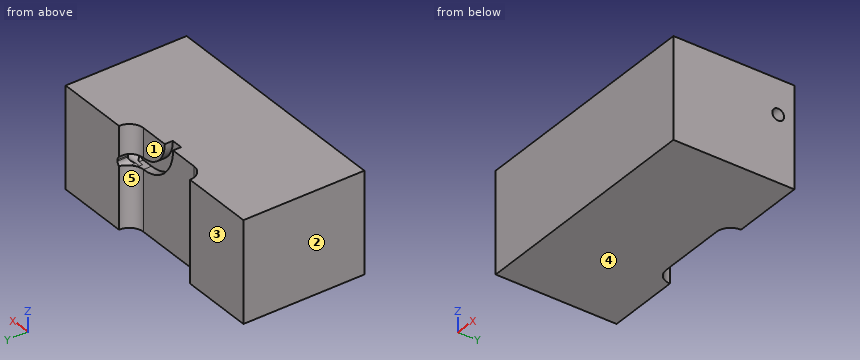
from build123d import *

# Parameters (mm, degrees)
SKETCH1_W               = 38.1
SKETCH1_H               = 15.875
BOSS_EXTRUDE1_DEPTH     = 19.05
CUT_EXTRUDE1_DEPTH      = 25.4
CUT_EXTRUDE2_DEPTH      = 27.62839016
CUT_EXTRUDE2_DEPTH_BACK = 1.27
SKETCH5_R               = 0.9271
CUT_EXTRUDE3_DEPTH      = 12.7


with BuildPart() as part:
    # Sketch1 → Boss-Extrude1 (new body)
    with BuildSketch(Plane(origin=(0, 0, 0), x_dir=(1, 0, 0), z_dir=(0, 1, 0))):
        Rectangle(SKETCH1_W, SKETCH1_H)
    extrude(amount=BOSS_EXTRUDE1_DEPTH)

    # Sketch2 → Cut-Extrude1 (cut)
    with BuildSketch(Plane(origin=(0, 0, -7.9375), x_dir=(-1, 0, 0), z_dir=(0, 0, -1))):
        with BuildLine():
            Line((5.3975, 16.8275), (-5.3975, 16.8275))
            ThreePointArc((-5.3975, 16.8275), (-7.62, 19.05), (-5.3975, 21.2725))
            Line((-5.3975, 21.2725), (5.3975, 21.2725))
            ThreePointArc((5.3975, 21.2725), (7.62, 19.05), (5.3975, 16.8275))
        make_face()
    extrude(amount=-CUT_EXTRUDE1_DEPTH, mode=Mode.SUBTRACT)

    # Sketch4 → Cut-Extrude2 (cut, two sides: drawn at the far end of the back side and taken through both)
    with BuildSketch(Plane(origin=(0, 16.8275, 0), x_dir=(1, 0, 0), z_dir=(0, 1, 0)).offset(-CUT_EXTRUDE2_DEPTH_BACK)):
        with BuildLine():
            Line((0.8255, -7.9375), (-0.9525, -7.9375))
            ThreePointArc((-0.9525, -7.9375), (0.907371939, -3.447371939), (5.3975, -1.5875))
            Line((5.3975, -1.5875), (7.14375, -1.5875))
            ThreePointArc((7.14375, -1.5875), (7.705016008, -1.819983992), (7.9375, -2.38125))
            Line((7.9375, -2.38125), (7.9375, -2.57175))
            ThreePointArc((7.9375, -2.57175), (7.705016008, -3.133016008), (7.14375, -3.3655))
            Line((7.14375, -3.3655), (5.3975, -3.3655))
            ThreePointArc((5.3975, -3.3655), (2.164607796, -4.704607796), (0.8255, -7.9375))
        make_face()
    extrude(amount=CUT_EXTRUDE2_DEPTH + CUT_EXTRUDE2_DEPTH_BACK, mode=Mode.SUBTRACT)

    # Sketch5 → Cut-Extrude3 (cut)
    with BuildSketch(Plane(origin=(19.05, 0, 0), x_dir=(0, 0, -1), z_dir=(1, 0, 0))):
        with Locations((-2.4765, 16.51)):
            Circle(SKETCH5_R)
    extrude(amount=-CUT_EXTRUDE3_DEPTH, mode=Mode.SUBTRACT)


solid = part.part
Geometry check sheet. Reference: the model listing, model coordinates, mm. Face numbers are marked on the shaded views. A direction names the side the tool comes from. Round coordinates to 2 decimals unless told otherwise and drop trailing zeros. Answer in a Markdown table with one row per item. Add a question column.
Item 1: Depth check by flat-ended pin: pin 1 Ø7 at (x, z) = (2.5, 5.5) entering from +Y; pin 2 Ø1.4 at (x, z) = (2.5, 5) entering from +Y. Enter the tip coordinate at first touch or a pass-through.
Item 2: Material ranges on L1, parallel to Z at x = 12, y = 16.51; L2, parallel to Y at x = 0, z = -1.25; L3, parallel to Y at x = 4, z = 3, recorded low to high. Write a range as [from, to].
Item 3: Draft check along X on the marked faces 1, 2 and 3. Enter one of: released by +X, released by -X, zero draft, split by the parting line, or undercut.
Item 4: Set-up check for the marked faces 4 and 5: record each of +Z, -Z, +X, -X, +Y, -Y from which the full face is reachable in a straight line by a thin tool's end or side.
Filled in:
| question | item | result |
|---|---|---|
| 1 | pin 1 | stops at y = 16.91 |
| 1 | pin 2 | stops at y = 16.83 |
| 2 | L1 | z = [-7.94, 1.55], [3.4, 7.94] |
| 2 | L2 | y = [0, 16.83] |
| 2 | L3 | y = [0, 15.56] |
| 3 | face 1 | undercut |
| 3 | face 2 | released by -X |
| 3 | face 3 | zero draft |
| 4 | face 4 | -Z, +X, -X, +Y, -Y |
| 4 | face 5 | +Z, -Z, +Y |
